The model under review builds one solid part; all positions refer to its coordinate system, in mm. Coordinates: 2 decimals unless noted, no trailing zeros. Order: outer loops, then holes, each group sorted by start corner. A loop starts at its lowest first (then second) coordinate and runs counter-clockwise, first axis right, second up. Notation, with made-up numbers: M -5,-10 L 9,-10 A15 ccw 9,13 Z; hole C 47.5,84 d3. An arc over 180 degrees is marked long. Answer in a Markdown table with one row per item.
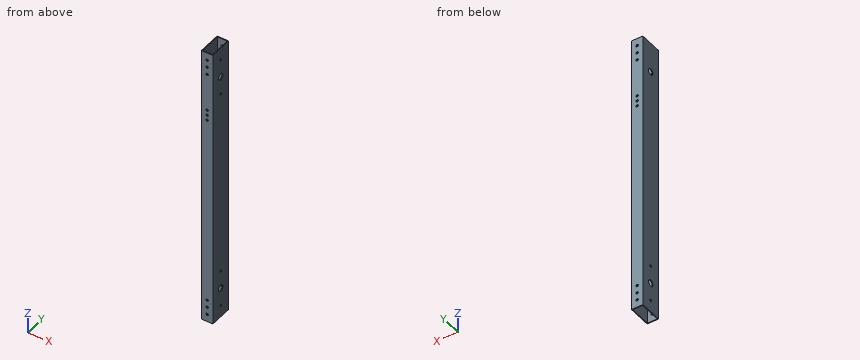
Autodesk Inventor part; units mm, degrees
ref_plane "YZ Plane" through (0, 0, 0) normal (1, 0, 0) x (0, 1, 0)
ref_plane "XZ Plane" through (0, 0, 0) normal (0, 1, 0) x (-1, 0, 0)
ref_plane "XY Plane" through (0, 0, 0) normal (0, 0, 1) x (1, 0, 0)
sketch "スケッチ1" plane through (0, 0, 0) normal (0, 0, 1) x (1, 0, 0)
  line L0 (0, 0) -> (15, 0)
  line L1 (15, 0) -> (15, 30)
  line L2 (15, 30) -> (0, 30)
  line L3 (0, 30) -> (0, 0)
  line L4 (1, 1) -> (14, 1)
  line L5 (14, 1) -> (14, 29)
  line L6 (14, 29) -> (1, 29)
  line L7 (1, 29) -> (1, 1)
  dimension "d0" = 15
  dimension "d1" = 30
  dimension "d2" = 13
  dimension "d3" = 28
  dimension "d4" = 1
  dimension "d5" = 1
extrude "押し出し1" add sketch "スケッチ1" along normal blind 375
sketch "スケッチ2" plane through (0, 30, 0) normal (0, 1, 0) x (1, 0, 0)
  circle A0 centre (7.5, -295) radius 1.6
  line L0 (0, 0) -> (0, -375)
  line L1 (15, -375) -> (0, -375)
  circle A1 centre (7.5, -302) radius 1.6
  circle A2 centre (7.5, -288) radius 1.6
  dimension "d8" = 3.2
  dimension "d9" = 7.5
  dimension "d10" = 80
  dimension "d11" = 3.2
  dimension "d12" = 3.2
  dimension "d13" = 7
  dimension "d14" = 7
hole "穴1" at (7.5, 30, 302) at (7.5, 30, 295) at (7.5, 30, 288) direction (0, -1, 0) diameter 3.2 depth 30
sketch "スケッチ3" plane through (0, 30, 0) normal (0, 1, 0) x (1, 0, 0)
  circle A0 centre (7.5, -10) radius 1.6
  line L0 (15, 0) -> (0, 0)
  line L1 (15, 0) -> (15, -375)
  circle A1 centre (7.5, -20) radius 1.6
  circle A2 centre (7.5, -30) radius 1.6
  line L2 (15, -187.5) -> (0, -187.5) construction
  line L3 (0, 0) -> (0, -375)
  line L4 (15, -375) -> (0, -375)
  circle A3 centre (7.5, -365) radius 1.6
  circle A4 centre (7.5, -355) radius 1.6
  circle A5 centre (7.5, -345) radius 1.6
  dimension "d22" = 3.2
  dimension "d23" = 10
  dimension "d24" = 7.5
  dimension "d25" = 3.2
  dimension "d26" = 3.2
  dimension "d27" = 10
  dimension "d28" = 7.5
  dimension "d29" = 10
  dimension "d30" = 7.5
  dimension "d31" = 187.5
hole "穴2" at (7.5, 30, 365) at (7.5, 30, 355) at (7.5, 30, 345) at (7.5, 30, 30) at (7.5, 30, 20) at (7.5, 30, 10) direction (0, -1, 0) diameter 3.2 depth 30
sketch "スケッチ4" plane through (0, 30, 0) normal (0, 1, 0) x (1, 0, 0)
  circle A0 centre (7.5, -302) radius 1.6
  line L0 (15, 0) -> (15, -375)
  line L1 (15, -375) -> (0, -375)
  line L2 (15, 0) -> (15, -375)
  line L3 (15, -187.5) -> (0, -187.5) construction
  line L4 (0, 0) -> (0, -375)
  dimension "d39" = 3.2
  dimension "d40" = 7.5
  dimension "d41" = 73
  dimension "d42" = 187.5
extrude "押し出し2" add sketch "スケッチ4" against normal blind 1
sketch "スケッチ5" plane through (0, 0, 0) normal (0, -1, 0) x (1, 0, 0)
  point P0 (0, 0)
sketch "スケッチ6" plane through (0, 0, 0) normal (0, -1, 0) x (1, 0, 0)
  circle A0 centre (7.5, 302) radius 1.6
  line L0 (15, 0) -> (15, 375)
  line L1 (0, 375) -> (15, 375)
  point P0 (0, 0)
  dimension "d45" = 3.2
  dimension "d46" = 7.5
  dimension "d47" = 73
extrude "押し出し3" add sketch "スケッチ6" against normal blind 1
sketch "スケッチ7" plane through (0, 30, 0) normal (0, 1, 0) x (1, 0, 0)
  circle A0 centre (7.5, -281) radius 1.6
  circle A1 centre (7.5, -288) radius 1.6
  line L0 (0, 0) -> (0, -375)
  dimension "d50" = 3.2
  dimension "d51" = 7
  dimension "d52" = 7.5
extrude "押し出し4" cut sketch "スケッチ7" against normal blind 30 contours A0
sketch "スケッチ8" plane through (15, 0, 0) normal (1, 0, 0) x (0, 0, -1)
  circle A0 centre (-335, 15) radius 4.25
  line L0 (0, 30) -> (-375, 30)
  line L1 (-375, 0) -> (-375, 30)
  point P0 (0, 0)
  dimension "d55" = 8.5
  dimension "d56" = 15
  dimension "d57" = 40
extrude "押し出し5" cut sketch "スケッチ8" against normal blind 30
sketch "スケッチ9" plane through (15, 0, 0) normal (1, 0, 0) x (0, 0, -1)
  circle A0 centre (-359, 15) radius 1.6
  line L0 (0, 30) -> (-375, 30)
  line L1 (-375, 0) -> (-375, 30)
  line L2 (-335, 0) -> (-335, 30) construction
  circle A1 centre (-311, 15) radius 1.6
  point P0 (0, 0)
  dimension "d60" = 3.2
  dimension "d61" = 15
  dimension "d62" = 16
  dimension "d63" = 40
hole "穴3" at (15, 15, 359) at (15, 15, 311) direction (-1, 0, 0) diameter 3.2 depth 5
sketch "スケッチ10" plane through (15, 0, 0) normal (1, 0, 0) x (0, 0, -1)
  circle A0 centre (-40, 15) radius 4.25
  line L0 (0, 0) -> (0, 30)
  line L1 (0, 30) -> (-375, 30)
  dimension "d71" = 8.5
  dimension "d72" = 40
  dimension "d73" = 15
extrude "押し出し6" cut sketch "スケッチ10" against normal blind 30
sketch "スケッチ11" plane through (15, 0, 0) normal (1, 0, 0) x (0, 0, -1)
  circle A0 centre (-64, 15) radius 1.6
  line L0 (0, 0) -> (0, 30)
  line L1 (0, 30) -> (-375, 30)
  circle A1 centre (-16, 15) radius 1.6
  circle A2 centre (-40, 15) radius 4.25
  line L2 (0, 0) -> (-375, 0)
  dimension "d76" = 3.2
  dimension "d77" = 64
  dimension "d78" = 15
  dimension "d79" = 3.2
  dimension "d80" = 24
  dimension "d81" = 15
hole "穴4" at (15, 15, 64) at (15, 15, 16) direction (-1, 0, 0) diameter 3.2 depth 15
equation "\"BendRadius\" = Thickness"
equation "\"BendReliefWidth\" = Thickness"
equation "\"BendReliefDepth\" = 0.5 * Thickness"
equation "\"CornerReliefSize\" = 4 * Thickness"
equation "\"MinimumRemnant\" = 2 * Thickness"
equation "\"TransitionRadius\" = BendRadius"
equation "\"JacobiRadiusSize\" = BendRadius"
equation "\"GapSize\" = Thickness"
properties part number "nhk43"
(1) Insertion check: P1, Ø2.5, axis at x = 7.5, z = 288, coming from the -Y side. The pin has a flat end and moves straight along its axis. Give the tip position at first contact, or say it passes through.
Report:
| item | result |
|---|---|
| P1 | through |
(2) Take a section at B-B (z = 40). Write out the cut boundary in (x, y).
Report:
| item | result |
|---|---|
| outline | M 0,0 L 15,0 L 15,10.75 L 14,10.75 L 14,1 L 1,1 L 1,10.75 L 0,10.75 Z; M 0,19.25 L 1,19.25 L 1,29 L 14,29 L 14,19.25 L 15,19.25 L 15,30 L 0,30 Z |
(3) Take a section at C-C (z = 86.5). Write out the cut boundary in (x, y), then the cut area to 3 significant figures.
Report:
| item | result |
|---|---|
| outline | M 0,0 L 15,0 L 15,30 L 0,30 Z; hole M 1,1 L 14,1 L 14,29 L 1,29 Z |
| area | 86.0 mm^2 |
(4) Take a section at A-A (y = 22.75). Write out the cut boundary in (x, z), then the cut area to 3 significant figures.
Report:
| item | result |
|---|---|
| outline | M 0,0 L 1,0 L 1,375 L 0,375 Z; M 14,0 L 15,0 L 15,375 L 14,375 Z |
| area | 750 mm^2 |
(5) To check wall thickness, follow line 1 (Y direction, x = 1.5, z = 156.5); line 2 (X direction, y = 22.5, z = 265); line 3 (Y direction, x = 14.5, z = 311). State the ranges of each line that lie inside material, in increasing order. Write a range as [from, to].
Report:
| item | result |
|---|---|
| line 1 | [0, 1], [29, 30] |
| line 2 | [0, 1], [14, 15] |
| line 3 | [0, 13.4], [16.6, 30] |
